from build123d import *

# Parameters (mm, degrees)
F0_R     = 31.25
F0_R_2   = 16
F1_DEPTH = 90
F0_R_3   = 46.875
F2_DEPTH = 60
F0_R_4   = 62.5
F3_DEPTH = 30
F4_R     = 50
F4_R_2   = 20
F5_DEPTH = 25


with BuildPart() as f1:
    # F0 (on Front) → F1 (new body)
    with BuildSketch(Plane.XZ):
        Circle(F0_R)
        Circle(F0_R_2, mode=Mode.SUBTRACT)
    extrude(amount=F1_DEPTH)

    # F0 (on Front) → F2 (join)
    with BuildSketch(Plane.XZ):
        Circle(F0_R_3)
        Circle(F0_R, mode=Mode.SUBTRACT)
    extrude(amount=F2_DEPTH)

    # F0 (on Front) → F3 (join)
    with BuildSketch(Plane.XZ):
        Circle(F0_R_4)
        Circle(F0_R_3, mode=Mode.SUBTRACT)
    extrude(amount=F3_DEPTH)

    # F4 (on Front) → F5 (cut)
    with BuildSketch(Plane.XZ):
        Circle(F4_R)
        Circle(F4_R_2, mode=Mode.SUBTRACT)
    extrude(amount=F5_DEPTH, mode=Mode.SUBTRACT)


solid = f1.part
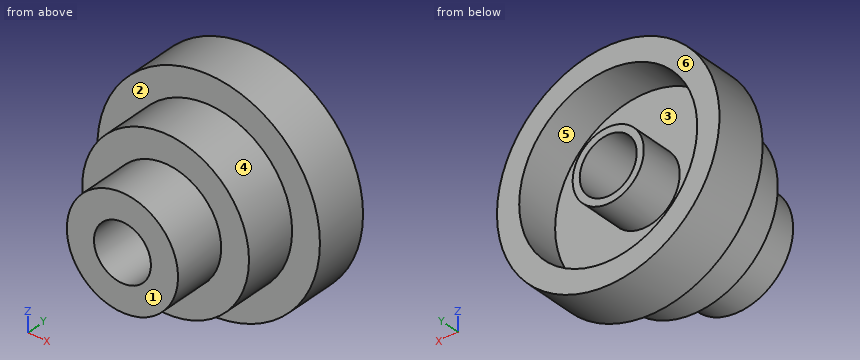
CAD build for the part. Positions are in the model's coordinates, mm. Face numbers are marked on the shaded views. A direction names the side the tool comes from. Round coordinates to 2 decimals unless told otherwise and drop trailing zeros. Write each loop counter-clockwise with the first axis right and the second up, starting at its lowest first coordinate (ties: lowest second). Pieces come first, ordered by that corner, then holes. Notation, with made-up numbers: M 7,65 L 19,65 A14 cw 19,84 Z; hole C -21,10 d5. An arc over 180 degrees is marked long. Use a Markdown table: item, result. Add a question column.
1. Slice it at D-D on z = -24.5. Give the cut face in (x, y).
2. Slice it at B-B on x = 0. Give the cut face in (y, z) (3 decimals).
3. Drill centre lines: probe 1 along Z at (x, y) = (0, -19.5); probe 2 along Z at (x, y) = (0, -50.5) (3 decimals); probe 3 along X at (y, z) = (-19.5, -7) (1 decimal). Where is each one in solid material? Low to high.
4. Flat gauge pins, fed straight in: P1, Ø1, axis at y = -76.5, z = 12, coming from the -X side; P2, Ø5, axis at x = -27.5, z = 1.5, coming from the +Y side; P3, Ø4, axis at x = -48, z = -13, coming from the -Y side. Where does each tip first touch, or does it go through?
5. 3-axis set-ups, long thin cutter, end or side, ignore diameter. For the marked faces 1, 2 and 3: which of +Z, -Z, +X, -X, +Y, -Y reach the whole face in a straight line?
6. Slice it at C-C on y = -27.5. Give the cut face in (x, z).
7. Slice it at A-A on z = 0. Give the cut face in (x, y) (3 decimals), then the cut area to 3 significant figures.
8. Pull direction Z, two halves, no side cores. Call the marked faces 4, 5 and 6: released by +Z, released by -Z, zero draft, split by the parting line, or undercut.
Reply:
| question | item | result |
|---|---|---|
| 1 | outline | M -57.5,-30 L -39.96,-30 L -39.96,-60 L -19.4,-60 L -19.4,-90 L 19.4,-90 L 19.4,-60 L 39.96,-60 L 39.96,-30 L 57.5,-30 L 57.5,0 L 43.59,0 L 43.59,-25 L -43.59,-25 L -43.59,0 L -57.5,0 Z |
| 2 | outline | M -90,-31.25 L -60,-31.25 L -60,-46.875 L -30,-46.875 L -30,-62.5 L 0,-62.5 L 0,-50 L -25,-50 L -25,-20 L 0,-20 L 0,-16 L -90,-16 Z; M -90,16 L 0,16 L 0,20 L -25,20 L -25,50 L 0,50 L 0,62.5 L -30,62.5 L -30,46.875 L -60,46.875 L -60,31.25 L -90,31.25 Z |
| 3 | probe 1 | z = -62.5 to -50, -20 to -16, 16 to 20, 50 to 62.5 |
| 3 | probe 2 | z = -46.875 to -16, 16 to 46.875 |
| 3 | probe 3 | x = -62.1 to -49.5, -18.7 to -14.4, 14.4 to 18.7, 49.5 to 62.1 |
| 4 | P1 | stops at x = -29.06 |
| 4 | P2 | stops at y = -25 |
| 4 | P3 | stops at y = -30 |
| 5 | face 1 | +Z, -Z, +X, -X, -Y |
| 5 | face 2 | -Y |
| 5 | face 3 | +Y |
| 6 | outline | C 0,0 d125; hole C 0,0 d32 |
| 7 | outline | M -62.5,-30 L -46.875,-30 L -46.875,-60 L -31.25,-60 L -31.25,-90 L -16,-90 L -16,0 L -20,0 L -20,-25 L -50,-25 L -50,0 L -62.5,0 Z; M 16,-90 L 31.25,-90 L 31.25,-60 L 46.875,-60 L 46.875,-30 L 62.5,-30 L 62.5,0 L 50,0 L 50,-25 L 20,-25 L 20,0 L 16,0 Z |
| 7 | area | 4,060 mm^2 |
| 8 | face 4 | split by the parting line |
| 8 | face 5 | undercut |
| 8 | face 6 | zero draft |
